```python
from build123d import *

# Parameters (mm, degrees)
F0_R     = 34.925
F1_DEPTH = 6.35
F3_DEPTH = 3.175


with BuildPart() as f1:
    # F0 (on Front) → F1 (new body, symmetric)
    with BuildSketch(Plane.XZ):
        Polygon((27.8911357684, 27.8911357684), (10.2088642316, 38.1), (-10.2088642316, 38.1), (-27.8911357684, 27.8911357684), (-38.1, 10.2088642316), (-38.1, -10.2088642316), (-27.8911357684, -27.8911357684), (-10.2088642316, -38.1), (10.2088642316, -38.1), (27.8911357684, -27.8911357684), (38.1, -10.2088642316), (38.1, 10.2088642316), align=None)
        Circle(F0_R, mode=Mode.SUBTRACT)
    extrude(amount=F1_DEPTH, both=True)

    # F2 (on Front) → F3 (join, symmetric)
    with BuildSketch(Plane.XZ):
        with BuildLine():
            Line((-3.175, 28.3980633142), (-3.175, 34.7803824016))
            ThreePointArc((-3.175, 34.7803824016), (0, -34.925), (3.175, 34.7803824016))
            Line((3.175, 34.7803824016), (3.175, 28.3980633142))
            ThreePointArc((3.175, 28.3980633142), (0, -28.575), (-3.175, 28.3980633142))
        make_face()
    extrude(amount=F3_DEPTH, both=True)


solid = f1.part
```
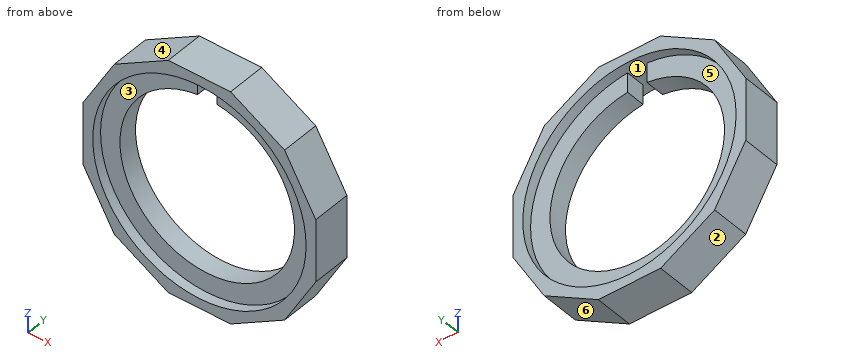
Could you check a few things on this model? Use its own coordinates, in mm. Face numbers are marked on the shaded views. A direction names the side the tool comes from. Give positions to 0.01 mm unless a question says otherwise; leave off trailing zeros. Loops run counter-clockwise (first coordinate to the right, second up) from the corner with the lowest first, then second, coordinate; pieces in that order, holes last. Notation, with made-up numbers: (25.5, 51) -> (59.5, 51) arc R22 cw to (59.5, 83) -> close; hole circle Ø1 at (-18.75, 54). An arc over 180 degrees is marked (long way). Put each result on its own line as item: value.
(1) For the marked faces 1, 2 and 3, which set-ups out of +Z, -Z, +X, -X, +Y, -Y let a thin tool reach every point of the face, with its end or its side?
Computed:
face 1: none
face 2: -Z, -X, +Y, -Y
face 3: -Y
(2) I'm going to push flat-ended pins straight in: pin 1 Ø3 at (y, z) = (0.5, -22.5) entering from -X; pin 2 Ø3 at (y, z) = (0.5, 33) entering from -X; pin 3 Ø2 at (x, z) = (-13.5, 29) entering from +Y (3 decimals); pin 4 Ø5 at (y, z) = (-1.5, -10.5) entering from +X. Where does each tip first touch, or does it pass through?
Computed:
pin 1: x = -31.87
pin 2: x = -21.64
pin 3: y = 3.175
pin 4: x = 38.1
(3) Please list where these lines run through material, in increasing order: probe 1 along X at (y, z) = (-1.5, 0) (3 decimals); probe 2 along Z at (x, y) = (0, 0.5) (3 decimals); probe 3 along Y at (x, z) = (31, 0.5) (3 decimals). Write a range as [from, to].
Computed:
probe 1: [-38.1, -28.575], [28.575, 38.1]
probe 2: [-38.1, -28.575], [34.925, 38.1]
probe 3: [-3.175, 3.175]
(4) Imagine slicing it at C-C on y = 1.25. Write out the boundary of the cut face in (x, z) (3 decimals), plus the area to 3 significant figures.
Computed:
outline: (-38.1, -10.209) -> (-27.891, -27.891) -> (-10.209, -38.1) -> (10.209, -38.1) -> (27.891, -27.891) -> (38.1, -10.209) -> (38.1, 10.209) -> (27.891, 27.891) -> (10.209, 38.1) -> (-10.209, 38.1) -> (-27.891, 27.891) -> (-38.1, 10.209) -> close; hole (-3.175, 28.398) arc R28.575 ccw (long way) to (3.175, 28.398) -> (3.175, 34.78) arc R34.925 ccw to (-3.175, 34.78) -> close
area: 2,060 mm^2
(5) Imagine slicing it at A-A on x = 0. Write out the boundary of the cut face in (y, z) (3 decimals), plus the area to 3 significant figures.
Computed:
outline: (-6.35, -38.1) -> (6.35, -38.1) -> (6.35, -34.925) -> (3.175, -34.925) -> (3.175, -28.575) -> (-3.175, -28.575) -> (-3.175, -34.925) -> (-6.35, -34.925) -> close; (-6.35, 34.925) -> (6.35, 34.925) -> (6.35, 38.1) -> (-6.35, 38.1) -> close
area: 121 mm^2
(6) Imagine slicing it at B-B on z = 0. Write out the boundary of the cut face in (x, y) (3 decimals), plus the area to 3 significant figures.
Computed:
outline: (-38.1, -6.35) -> (-34.925, -6.35) -> (-34.925, -3.175) -> (-28.575, -3.175) -> (-28.575, 3.175) -> (-34.925, 3.175) -> (-34.925, 6.35) -> (-38.1, 6.35) -> close; (28.575, -3.175) -> (34.925, -3.175) -> (34.925, -6.35) -> (38.1, -6.35) -> (38.1, 6.35) -> (34.925, 6.35) -> (34.925, 3.175) -> (28.575, 3.175) -> close
area: 161 mm^2
(7) Thinking about a two-plate mould opening in X: for the marked faces 4, 5 and 6, which applies, pulls with the +X half, pulls with the -X half, needs draft (parallel to the pull), parting line crosses it, or undercut?
Computed:
face 4: pulls with the -X half
face 5: undercut
face 6: pulls with the +X half
